Source: three-view drawing plus pictorial views. Frame: mm from the lowest corner of the part. A direction names the side the tool comes from. Give positions to 0.01 mm unless a question says otherwise; leave off trailing zeros. Write each loop counter-clockwise with the first axis right and the second up, starting at its lowest first coordinate (ties: lowest second). Pieces come first, ordered by that corner, then holes. Notation, with made-up numbers: (42, 47.25) -> (62, 47.25) arc R19 ccw to (62, 72.25) -> close; hole circle Ø3 at (41, -10.75). An arc over 180 degrees is marked (long way). Write item = value, one per line.
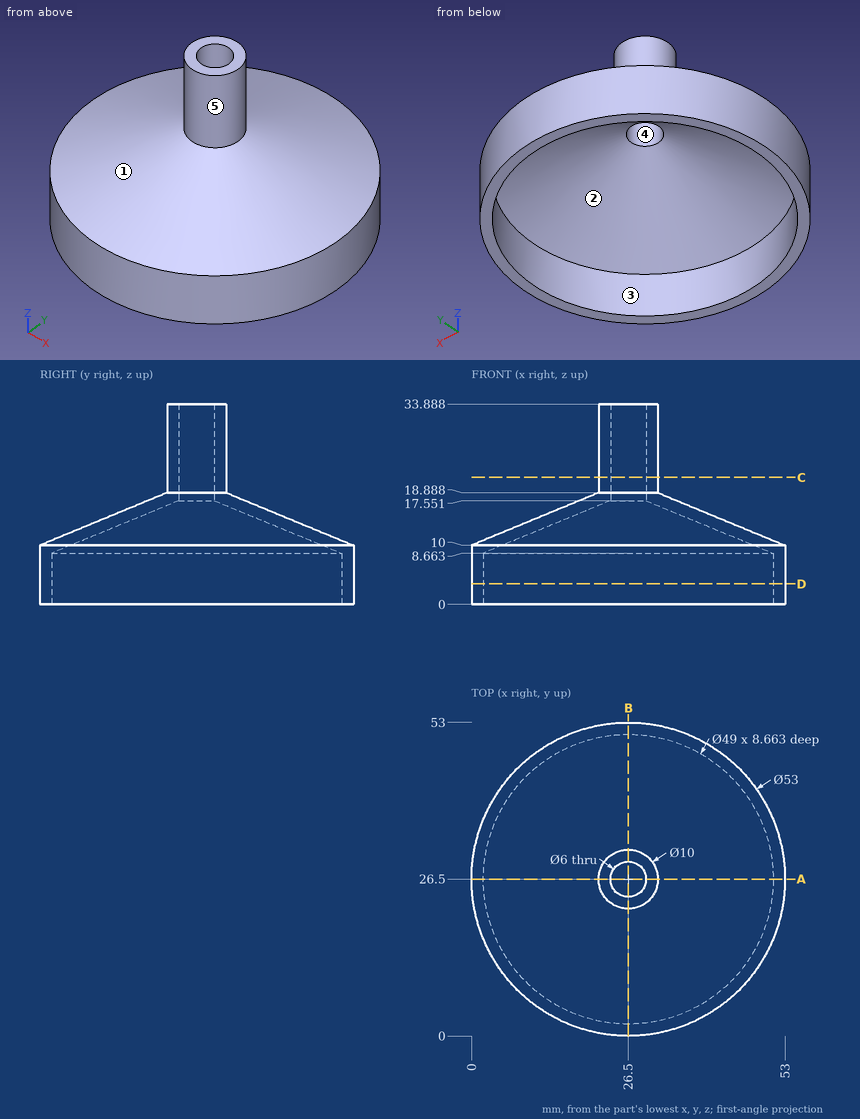
1) Draft query along X for the marked faces 1 and 2. Return one class per face: pulls with the +X half, pulls with the -X half, needs draft (parallel to the pull), parting line crosses it, or undercut.
Computed:
face_1 = parting line crosses it
face_2 = undercut
2) Access query for the marked faces 3, 4 and 5. Directions: +Z, -Z, +X, -X, +Y, -Y. A direction counts if a zero-diameter tool reaches every point of the face in a straight line with its end or side. Return the directions, or none.
Computed:
face_3 = -Z
face_4 = +Z, -Z
face_5 = +Z
3) Cut plane D-D (z = 3.5). Return the cut outline in (x, y).
Computed:
outline = circle Ø53 at (26.5, 26.5); hole circle Ø49 at (26.5, 26.5)
4) Cut plane C-C (z = 21.5). Return the cut outline in (x, y).
Computed:
outline = circle Ø10 at (26.5, 26.5); hole circle Ø6 at (26.5, 26.5)
5) Material intervals for L1, parallel to X at y = 26.5, z = 27; L2, parallel to X at y = 26, z = 6 (1 decimal), sorted ascending.
Computed:
L1 = 21.5 to 23.5, 29.5 to 31.5
L2 = 0 to 2, 51 to 53
6) Cut plane A-A (y = 26.5). Return the cut outline in (x, z).
Computed:
outline = (0, 0) -> (2, 0) -> (2, 8.66) -> (23.5, 17.55) -> (23.5, 33.89) -> (21.5, 33.89) -> (21.5, 18.89) -> (0, 10) -> close; (29.5, 17.55) -> (51, 8.66) -> (51, 0) -> (53, 0) -> (53, 10) -> (31.5, 18.89) -> (31.5, 33.89) -> (29.5, 33.89) -> close
7) Contact query for flat-ended pins moving along their axis: pin 1 (1.5 mm diameter, centred on x = 38, y = 42, fed in from +Z); pin 2 (2 mm diameter, centred on x = 24.5, y = 45.5, fed in from +Z); pin 3 (6 mm diameter, centred on x = 28.5, y = 10, fed in from +Z) (1 decimal). Output: stop coordinate, or through.
Computed:
pin_1 = 13.29
pin_2 = 13.47
pin_3 = 15.3
